Check sheet for the drawn part. Datum: minimum x, y, z corner. Units: mm. A direction names the side the tool comes from. Round coordinates to 2 decimals unless told otherwise and drop trailing zeros. Order: outer loops, then holes, each group sorted by start corner. A loop starts at its lowest first (then second) coordinate and runs counter-clockwise, first axis right, second up. Notation, with made-up numbers: (44.5, 62.25) -> (78.5, 62.25) arc R35 ccw to (78.5, 99.25) -> close; hole circle Ø11 at (-39.5, -7.75). An arc over 180 degrees is marked (long way). Answer as a JSON object with one key per item and string values. Group by question number.
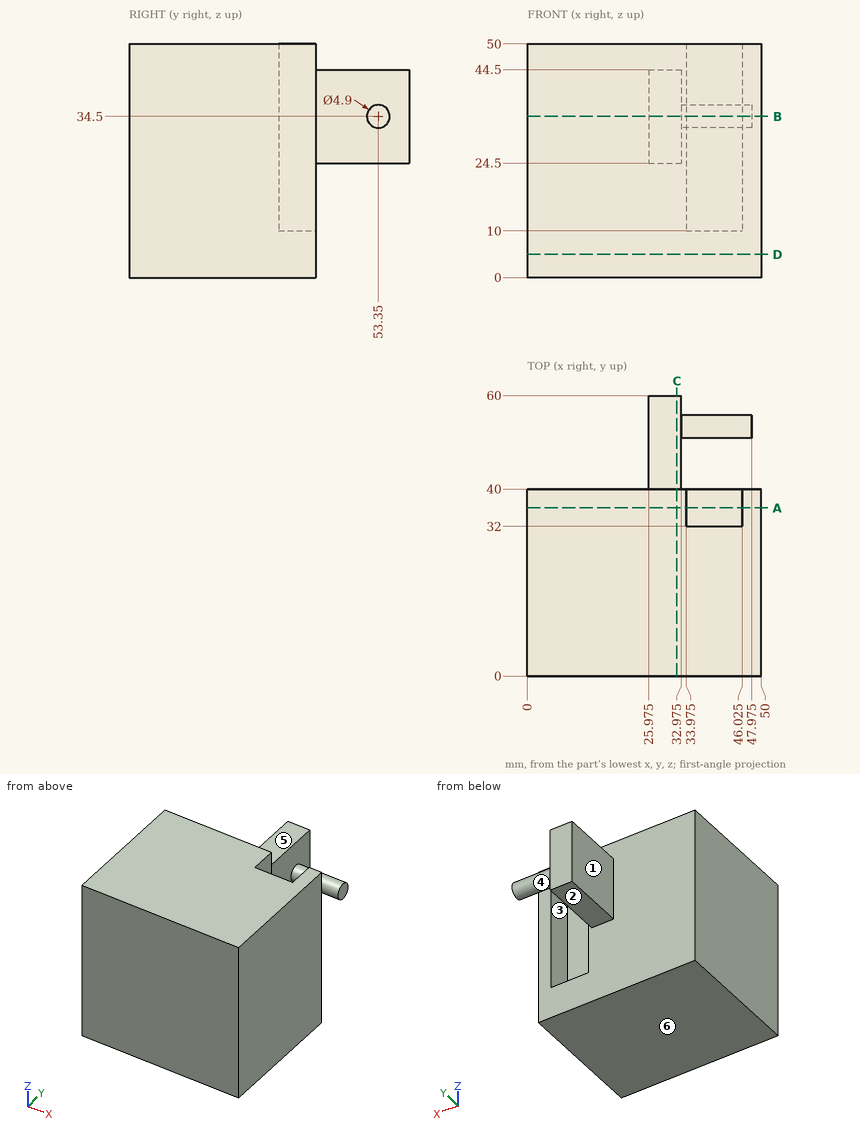
Item 1: Set-up check for the marked faces 4, 5 and 6: record each of +Z, -Z, +X, -X, +Y, -Y from which the full face is reachable in a straight line by a thin tool's end or side.
Item 2: Depth check by flat-ended pin: pin 1 Ø6 at (y, z) = (48.5, 38.5) entering from -X (3 decimals); pin 2 Ø1 at (x, z) = (36.5, 29) entering from +Y; pin 3 Ø5.5 at (y, z) = (54, 35.5) entering from +X (3 decimals). Enter the tip coordinate at first touch or a pass-through.
Item 3: Sectioned sample at A-A, the plane y = 36. Enter the section's corners in (x, z) (3 decimals).
Item 4: Mould release check, pull along X, two halves, no side actions. Record for the marked faces 1, 2 and 3: pulls with the +X half, pulls with the -X half, needs draft (parallel to the pull), parting line crosses it, or undercut.
Item 5: Thickness scan on L1, parallel to Y at x = 16, z = 10.5; L2, parallel to Y at x = 39.5, z = 27.5; L3, parallel to Z at x = 28, y = 45.5. Record the ranges inside material, lowest first.
Item 6: Sectioned sample at D-D, the plane z = 5. Enter the section's corners in (x, y), then the cut area to 3 significant figures.
Item 7: Sectioned sample at B-B, the plane z = 34.5. Enter the section's corners in (x, y) (3 decimals).
Item 8: Sectioned sample at C-C, the plane x = 32. Enter the section's corners in (y, z), then the cut area to 3 significant figures.
Result:
{
 "1": {"face 4": "+X", "face 5": "+Z, +X, -X, +Y", "face 6": "-Z, +X, -X, +Y, -Y"},
 "2": {"pin 1": "stops at x = 25.975", "pin 2": "stops at y = 32", "pin 3": "stops at x = 47.975"},
 "3": {"outline": "(0, 0) -> (50, 0) -> (50, 50) -> (46.025, 50) -> (46.025, 10) -> (33.975, 10) -> (33.975, 50) -> (0, 50) -> close"},
 "4": {"face 1": "pulls with the -X half", "face 2": "needs draft", "face 3": "undercut"},
 "5": {"L1": "y = 0 to 40", "L2": "y = 0 to 32", "L3": "z = 24.5 to 44.5"},
 "6": {"outline": "(0, 0) -> (50, 0) -> (50, 40) -> (0, 40) -> close", "area": "2,000 mm2"},
 "7": {"outline": "(0, 0) -> (50, 0) -> (50, 40) -> (46.025, 40) -> (46.025, 32) -> (33.975, 32) -> (33.975, 40) -> (32.975, 40) -> (32.975, 50.9) -> (47.975, 50.9) -> (47.975, 55.8) -> (32.975, 55.8) -> (32.975, 60) -> (25.975, 60) -> (25.975, 40) -> (0, 40) -> close"},
 "8": {"outline": "(0, 0) -> (40, 0) -> (40, 24.5) -> (60, 24.5) -> (60, 44.5) -> (40, 44.5) -> (40, 50) -> (0, 50) -> close", "area": "2,400 mm2"}
}
